from build123d import *

# Parameters (mm, degrees)
F0_R     = 2.2
F1_DEPTH = 15
F2_R     = 2.2
F3_DEPTH = 15


with BuildPart() as f1:
    # F0 (on Front) → F1 (new body)
    with BuildSketch(Plane.XZ):
        with BuildLine():
            Line((8.592964, -25.75), (25.75, -25.75))
            Line((25.75, -25.75), (25.75, 0))
            ThreePointArc((25.75, 0), (24.573215, 7.695427), (21.150419, 14.687487))
            Line((21.150419, 14.687487), (23.486593, 16.752013))
            ThreePointArc((23.486593, 16.752013), (23.747987, 20.986593), (19.513407, 21.247987))
            Line((19.513407, 21.247987), (17.177232, 19.183461))
            ThreePointArc((17.177232, 19.183461), (-10.505921, 23.50932), (-25.75, 0))
            ThreePointArc((-25.75, 0), (-24.545164, -7.667474), (-21.046787, -14.595905))
            Line((-21.046787, -14.595905), (-23.486593, -16.752013))
            ThreePointArc((-23.486593, -16.752013), (-23.747987, -20.986593), (-19.513407, -21.247987))
            Line((-19.513407, -21.247987), (-16.983615, -19.012358))
            ThreePointArc((-16.983615, -19.012358), (-4.7787, -24.673256), (8.592964, -23.188554))
            Line((8.592964, -23.188554), (8.592964, -25.75))
        make_face()
        with Locations((-21.5, -19)):
            Circle(F0_R, mode=Mode.SUBTRACT)
        with Locations((21.5, 19)):
            Circle(F0_R, mode=Mode.SUBTRACT)
    extrude(amount=F1_DEPTH)


with BuildPart() as f3:
    # F2 (on Front) → F3 (new body)
    with BuildSketch(Plane.XZ):
        Polygon((25.75, 14.25), (25.75, 24.25), (-26.25, 24.25), (-26.25, -25.75), (-16.25, -25.75), (-16.25, 14.25), align=None)
        with Locations((-21.5, -19)):
            Circle(F2_R, mode=Mode.SUBTRACT)
        with Locations((21.5, 19)):
            Circle(F2_R, mode=Mode.SUBTRACT)
    extrude(amount=-F3_DEPTH)


solid = f3.part
CAD build for the part. Positions are in the model's coordinates, mm. A direction names the side the tool comes from. Give positions to 0.01 mm unless a question says otherwise; leave off trailing zeros. Order: outer loops, then holes, each group sorted by start corner. A loop starts at its lowest first (then second) coordinate and runs counter-clockwise, first axis right, second up. Notation, with made-up numbers: (-15.5, 89) - (36.5, 89) arc R34 cw to (36.5, 126) - close; hole circle Ø8 at (71.25, -31.75). An arc over 180 degrees is marked (long way). Write each question's results on one line, items separated by ' | '.
1. Saw through at D-D on z = -1. List the corners of the cut face in (x, y), and give its area (3 significant figures).
Calculated:
outline: (-26.25, 0) - (-16.25, 0) - (-16.25, 15) - (-26.25, 15) - close | area: 150 mm2
2. Saw through at A-A on z = -19. List the corners of the cut face in (x, y), and give its area (3 significant figures).
Calculated:
outline: (-26.25, 0) - (-23.7, 0) - (-23.7, 15) - (-26.25, 15) - close; (-19.3, 0) - (-16.25, 0) - (-16.25, 15) - (-19.3, 15) - close | area: 84.0 mm2
3. Pin check, flat tips, straight feed: pin 1 (5 mm diameter, centred on y = 7.5, z = 6.5, fed in from +X); pin 2 (4 mm diameter, centred on x = -3.5, y = 12, fed in from -Z). Stop position of each tip, or through.
Calculated:
pin 1: stops at x = -16.25 | pin 2: stops at z = 14.25
4. Pull direction X, two halves, no side cores. Call faces 3 (the face through (-16.25, 7, -6)), 4 (the face through (-19.468, 7.395, -19.843)), 5 (the face through (-26.25, 7, 0)), 6 (the face through (0, 7, 24.25)): released by +X, released by -X, zero draft, split by the parting line, or undercut.
Calculated:
face 3: released by +X | face 4: undercut | face 5: released by -X | face 6: zero draft
5. Saw through at B-B on x = -21.5. List the corners of the cut face in (y, z).
Calculated:
outline: (0, -25.75) - (15, -25.75) - (15, -21.2) - (0, -21.2) - close; (0, -16.8) - (15, -16.8) - (15, 24.25) - (0, 24.25) - close
6. Probe L1, parallel to Z at x = 21.5, y = 10.75; L2, parallel to Z at x = -21.5, y = 4.25; L3, parallel to Z at x = -12, y = 2.5. List the from-to ranges inside material, lowest first. Write a range as from..to.
Calculated:
L1: z = 14.25..16.8, 21.2..24.25 | L2: z = -25.75..-21.2, -16.8..24.25 | L3: z = 14.25..24.25
7. 3-axis set-ups, long thin cutter, end or side, ignore diameter. For faces 1 (the face through (23.532, 7.395, 18.157)), 2 (the face through (4, 7, 14.25)): which of +Z, -Z, +X, -X, +Y, -Y reach the whole face in a straight line?
Calculated:
face 1: +Y, -Y | face 2: -Z, +X, +Y, -Y
8. Saw through at C-C on y = 2.25. List the corners of the cut face in (x, z), and give its area (3 significant figures).
Calculated:
outline: (-26.25, -25.75) - (-16.25, -25.75) - (-16.25, 14.25) - (25.75, 14.25) - (25.75, 24.25) - (-26.25, 24.25) - close; hole circle Ø4.4 at (-21.5, -19); hole circle Ø4.4 at (21.5, 19) | area: 890 mm2
